Verification items for the finished model (mm, model axes). A direction names the side the tool comes from. Coordinates: 2 decimals unless noted, no trailing zeros. Loops run counter-clockwise (first coordinate to the right, second up) from the corner with the lowest first, then second, coordinate; pieces in that order, holes last. Notation, with made-up numbers: M 84.5,-20 L 112.5,-20 A10 ccw 112.5,-7 Z; hole C -15,21.25 d7. An arc over 180 degrees is marked long. Write item = value, one per line. Start each with the question number.
```python
from build123d import *

# Parameters (mm, degrees)
F1_DEPTH = 30
F2_W     = 0.922354
F2_H     = 5.568772
F5_DEPTH = 13.899828
F3_W     = 3.941696
F3_H     = 5.368674
F6_DEPTH = 13.899828
F4_R     = 0.801782
F7_DEPTH = 13.899828


with BuildPart() as f1:
    # F0 (on Right) → F1 (new body, symmetric)
    with BuildSketch(Plane.YZ):
        with BuildLine():
            Line((3.898828, 10), (0, 10))
            Line((0, 10), (-3.898828, 10))
            Line((-3.898828, 10), (-3.898828, 0))
            ThreePointArc((-3.898828, 0), (0, -3.898828), (3.898828, 0))
            Line((3.898828, 0), (3.898828, 10))
        make_face()
    extrude(amount=F1_DEPTH, both=True)

    # F2 (on face) → F5 (cut, through all)
    with BuildSketch(Plane.XY.offset(10)):
        with Locations((-14.896151, 0)):
            Rectangle(F2_W, F2_H)
    extrude(amount=-F5_DEPTH, mode=Mode.SUBTRACT)

    # F3 (on face) → F6 (cut, through all)
    with BuildSketch(Plane.XY.offset(10)):
        with Locations((13.494484, 0)):
            Rectangle(F3_W, F3_H)
    extrude(amount=-F6_DEPTH, mode=Mode.SUBTRACT)

    # F4 (on face) → F7 (cut, through all)
    with BuildSketch(Plane.XY.offset(10)):
        with Locations((27.888514, 0)):
            Circle(F4_R)
    extrude(amount=-F7_DEPTH, mode=Mode.SUBTRACT)


solid = f1.part
```
Q1. Sectioned sample at B-B on z = 1.75. Record the cut outline in (x, y), plus the area to 3 significant figures.
Q2. Scan lines: L1, parallel to X at y = 1.25, z = 0; L2, parallel to X at y = 0, z = 6; L3, parallel to X at y = 0.5, z = 8.75. Record each from-to range of solid material in increasing order. Write a range as [from, to].
Q3. Sectioned sample at A-A on y = 0. Record the cut outline in (x, z), plus the area to 3 significant figures.
Q4. Mould release check, pull along Y, two halves, no side actions. Record for faces 3 (the face through (0, -3.899, 5)), 4 (the face through (0, 0, 10)), 5 (the face through (-15.357, 0, 3)), 6 (the face through (0.42, -0.086, -3.898)): +Y half, -Y half, draft (parallel to the pull), parting line (faces both ways), or undercut.
Q5. Gauge pin test, flat ends, axial feed: pin 1 (1.3 mm diameter, centred on x = 27.89, y = 0, fed in from -Z); pin 2 (1 mm diameter, centred on x = 23.5, y = 2, fed in from -Z); pin 3 (1.5 mm diameter, centred on x = -10, y = 1, fed in from -Z). Record the tip position at first contact, or that the pin passes through.
Q6. Sectioned sample at C-C on x = 17. Record the cut outline in (y, z).
Q7. Set-up check for faces 1 (the face through (0, 3.899, 5)), 2 (the face through (-14.435, 0, 3)): record each of +Z, -Z, +X, -X, +Y, -Y from which the full face is reachable in a straight line by a thin tool's end or side.
Solutions:
q1.outline = M -30,-3.9 L 30,-3.9 L 30,3.9 L -30,3.9 Z; hole M -15.36,-2.78 L -14.43,-2.78 L -14.43,2.78 L -15.36,2.78 Z; hole M 11.52,-2.68 L 15.47,-2.68 L 15.47,2.68 L 11.52,2.68 Z; hole C 27.89,0 d1.6
q1.area = 440 mm²
q2.L1 = [-30, -15.36], [-14.43, 11.52], [15.47, 30]
q2.L2 = [-30, -15.36], [-14.43, 11.52], [15.47, 27.09], [28.69, 30]
q2.L3 = [-30, -15.36], [-14.43, 11.52], [15.47, 27.26], [28.52, 30]
q3.outline = M -30,-3.9 L -15.36,-3.9 L -15.36,10 L -30,10 Z; M -14.43,-3.9 L 11.52,-3.9 L 11.52,10 L -14.43,10 Z; M 15.47,-3.9 L 27.09,-3.9 L 27.09,10 L 15.47,10 Z; M 28.69,-3.9 L 30,-3.9 L 30,10 L 28.69,10 Z
q3.area = 744 mm²
q4.face_3 = -Y half
q4.face_4 = draft
q4.face_5 = undercut
q4.face_6 = parting line
q5.pin_1 = through
q5.pin_2 = -3.6
q5.pin_3 = -3.89
q6.outline = M -3.9,0 A3.9 ccw 3.9,0 L 3.9,10 L -3.9,10 Z
q7.face_1 = +Z, -Z, +X, -X, +Y
q7.face_2 = +Z, -Z
